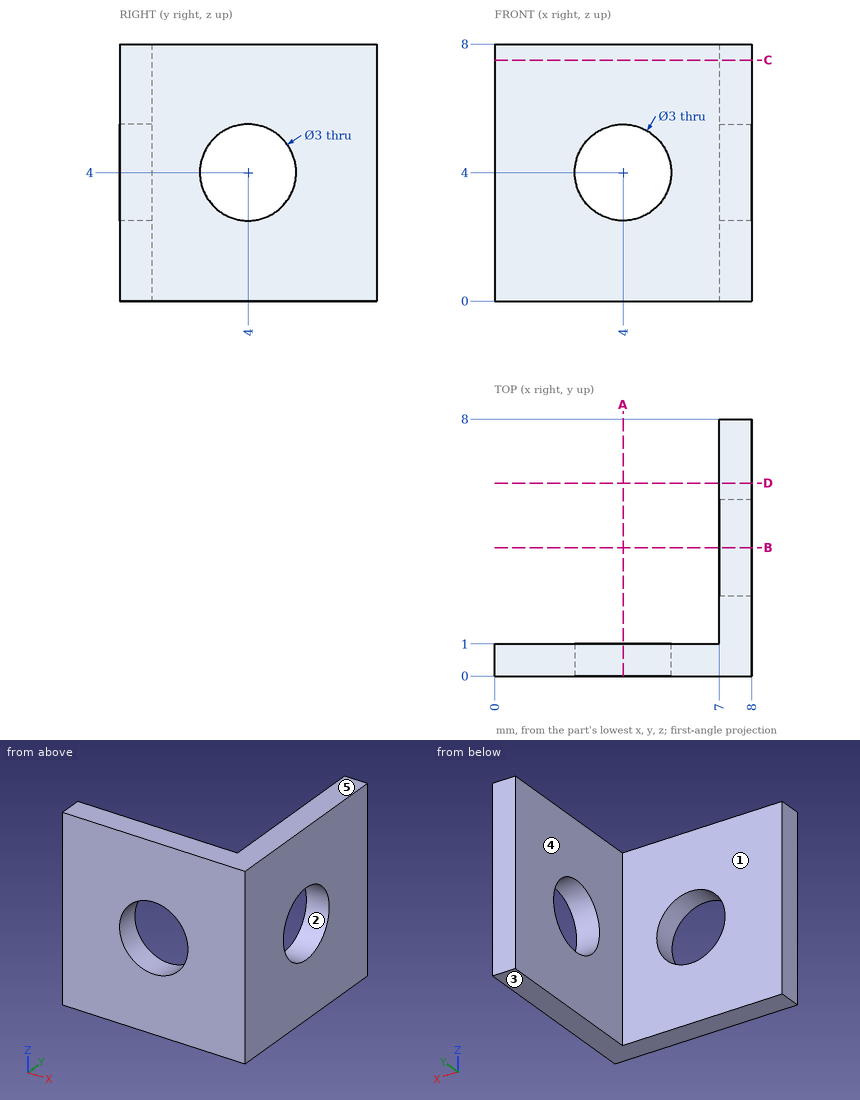
Design review of the part shown in the three views and the two pictorial views. Dimensions are in mm from the part's minimum x, y and z. A direction names the side the tool comes from. Round coordinates to 2 decimals unless told otherwise and drop trailing zeros. Loops run counter-clockwise (first coordinate to the right, second up) from the corner with the lowest first, then second, coordinate; pieces in that order, holes last. Notation, with made-up numbers: M -26.5,-14.75 L 5.5,-14.75 A26 ccw 5.5,15.25 Z; hole C 29,82.5 d7. An arc over 180 degrees is marked long. Put each result on its own line as item: value.
Q1. Mouldability with a two-part tool opening along Z and no side actions: class the marked faces 1, 2 and 3 as released by +Z, released by -Z, zero draft, split by the parting line, or undercut.
Result set:
face 1: zero draft
face 2: undercut
face 3: released by -Z
Q2. For pin 1 (4 mm diameter, centred on y = 4, z = 4, fed in from -X); pin 2 (2 mm diameter, centred on x = 2.5, z = 4.5, fed in from +Y); pin 3 (1.8 mm diameter, centred on x = 4, z = 4, fed in from -Y), all flat-tipped, find the tip position at first contact; note any pin that passes through.
Result set:
pin 1: stops at x = 7
pin 2: stops at y = 1
pin 3: passes through
Q3. Consider section D-D, the plane y = 6. Give the boundary of the cut face in (x, z), then the cut area to 3 significant figures.
Result set:
outline: M 7,0 L 8,0 L 8,8 L 7,8 Z
area: 8.00 mm²
Q4. Consider section B-B, the plane y = 4. Give the boundary of the cut face in (x, z).
Result set:
outline: M 7,0 L 8,0 L 8,2.5 L 7,2.5 Z; M 7,5.5 L 8,5.5 L 8,8 L 7,8 Z
Q5. Machinability: for the marked faces 4 and 5, which of the approach directions +Z, -Z, +X, -X, +Y, -Y give a long, thin tool a straight path to every point of the face, cutting with its end or side? Answer none if there is none.
Result set:
face 4: +Z, -Z, -X, +Y
face 5: +Z, +X, -X, +Y, -Y
Q6. Consider section A-A, the plane x = 4. Give the boundary of the cut face in (y, z).
Result set:
outline: M 0,0 L 1,0 L 1,2.5 L 0,2.5 Z; M 0,5.5 L 1,5.5 L 1,8 L 0,8 Z
Q7. Consider section C-C, the plane z = 7.5. Give the boundary of the cut face in (x, y).
Result set:
outline: M 0,0 L 8,0 L 8,8 L 7,8 L 7,1 L 0,1 Z
Q8. To check wall thickness, follow L1, parallel to Y at x = 7.55, z = 4; L2, parallel to Y at x = 2.5, z = 1. State the ranges of each line that lie inside material, in increasing order.
Result set:
L1: y = 0 to 2.5, 5.5 to 8
L2: y = 0 to 1
